```python
from build123d import *

# Parameters (mm, degrees)
SKETCH1_W             = 40
SKETCH1_H             = 30
BOSS_EXTRUDE1_DEPTH   = 6.35
SKETCH2_W             = 23.64
SKETCH2_H             = 6.35
CUT_EXTRUDE1_DEPTH    = 7.35
F_6_CLEARANCE_HOLE1_D = 3.6576


with BuildPart() as part:
    # Sketch1 → Boss-Extrude1 (new body)
    with BuildSketch(Plane(origin=(0, 0, 0), x_dir=(1, 0, 0), z_dir=(0, 1, 0))):
        Rectangle(SKETCH1_W, SKETCH1_H)
    extrude(amount=BOSS_EXTRUDE1_DEPTH)

    # Sketch2 → Cut-Extrude1 (cut, through all)
    with BuildSketch(Plane(origin=(0, 6.35, 0), x_dir=(1, 0, 0), z_dir=(0, 1, 0))):
        with Locations((0, 8.65)):
            Rectangle(SKETCH2_W, SKETCH2_H)
    extrude(amount=-CUT_EXTRUDE1_DEPTH, mode=Mode.SUBTRACT)

    # #6 Clearance Hole1 (through all)
    with Locations(Plane(origin=(0, 6.35, 0), x_dir=(1, 0, 0), z_dir=(0, 1, 0))):
        with Locations((0, -4.9898)):
            Hole(F_6_CLEARANCE_HOLE1_D / 2)


solid = part.part
```
Work out the finished part from the listing and answer in its coordinate system (mm). A direction names the side the tool comes from. Give positions to 0.01 mm unless a question says otherwise; leave off trailing zeros. Loops run counter-clockwise (first coordinate to the right, second up) from the corner with the lowest first, then second, coordinate; pieces in that order, holes last. Notation, with made-up numbers: (30.25, 85.5) -> (59.25, 85.5) arc R32 ccw to (59.25, 118.5) -> close; hole circle Ø5 at (-17, 82.25). An arc over 180 degrees is marked (long way). Put each result on its own line as item: value. Start each with the question number.
Item 1: Find the intervals of material crossed by L1, parallel to Z at x = 0, y = 2.5 (3 decimals); L2, parallel to Z at x = -4.5, y = 2 (3 decimals); L3, parallel to X at y = 3, z = 5, in increasing order. Write a range as [from, to].
Item 2: The part is cut by section D-D (y = 5.25). Give the vertices of the cut face in (x, z) (3 decimals), then the cut area to 3 significant figures.
Item 3: Which of the six approach directions +Z, -Z, +X, -X, +Y, -Y give full straight-line access (tool end or side, diameter ignored) to faces 1 (the face through (0, 0, 0)), 2 (the face through (0, 3, -5.475))?
Item 4: The part is cut by section B-B (z = -9.75). Give the vertices of the cut face in (x, y), then the cut area to 3 significant figures.
Item 5: The part is cut by section C-C (x = 5). Give the vertices of the cut face in (y, z) (3 decimals).
Item 6: The part is cut by section A-A (x = 0). Give the vertices of the cut face in (y, z) (3 decimals), then the cut area to 3 significant figures.
Item 7: The mould has two halves that part along Z. Classify faces 3 (the face through (-11.82, 3, -9)), 4 (the face through (20, 3, 0)), 5 (the face through (0, 3, 15)): released by +Z, released by -Z, zero draft, split by the parting line, or undercut.
Item 8: This flat-tipped pin is pushed along its axis until it touches: P1, Ø10, axis at x = 15, z = -5.5, coming from the -Y side. Where does it stop, or does it pass through?
Answers below:
1. L1: [-15, -11.825], [-5.475, 3.161], [6.819, 15]
1. L2: [-15, -11.825], [-5.475, 15]
1. L3: [-20, -1.83], [1.83, 20]
2. outline: (-20, -15) -> (20, -15) -> (20, 15) -> (-20, 15) -> close; hole (-11.82, -11.825) -> (11.82, -11.825) -> (11.82, -5.475) -> (-11.82, -5.475) -> close; hole circle Ø3.658 at (0, 4.99)
2. area: 1,040 mm2
3. face 1: +Z, -Z, +X, -X, -Y
3. face 2: +Y, -Y
4. outline: (-20, 0) -> (-11.82, 0) -> (-11.82, 6.35) -> (-20, 6.35) -> close; (11.82, 0) -> (20, 0) -> (20, 6.35) -> (11.82, 6.35) -> close
4. area: 104 mm2
5. outline: (0, -15) -> (6.35, -15) -> (6.35, -11.825) -> (0, -11.825) -> close; (0, -5.475) -> (6.35, -5.475) -> (6.35, 15) -> (0, 15) -> close
6. outline: (0, -15) -> (6.35, -15) -> (6.35, -11.825) -> (0, -11.825) -> close; (0, -5.475) -> (6.35, -5.475) -> (6.35, 3.161) -> (0, 3.161) -> close; (0, 6.819) -> (6.35, 6.819) -> (6.35, 15) -> (0, 15) -> close
6. area: 127 mm2
7. face 3: undercut
7. face 4: zero draft
7. face 5: released by +Z
8. P1: y = 0
